```python
from build123d import *

# Parameters (mm, degrees)
EXTRUDE_6_DEPTH      = 4
CUT_EXTRUDE_12_DEPTH = 3
SKETCH_3_R           = 2.6
CUT_EXTRUDE_13_DEPTH = 4


with BuildPart() as part:
    # 草圖1 → 填料-伸長6 (new body)
    with BuildSketch(Plane(origin=(0, 0, 0), x_dir=(1, 0, 0), z_dir=(0, 1, 0))):
        with BuildLine():
            Line((0, 0), (0, 38.27))
            ThreePointArc((0, 38.27), (10, 48.27), (20, 38.27))
            Line((20, 38.27), (20, 0))
            Line((20, 0), (0, 0))
        make_face()
    extrude(amount=-EXTRUDE_6_DEPTH)

    # 草圖2 → 除料-伸長12 (cut)
    with BuildSketch(Plane(origin=(0, 0, 0), x_dir=(1, 0, 0), z_dir=(0, 1, 0))):
        with BuildLine():
            Line((7.4, 38.722411537), (5, 24.929659817))
            ThreePointArc((5, 24.929659817), (3.500000254, 20.778165453), (4.997678036, 16.625832861))
            Line((4.997678036, 16.625832861), (7.4, 2.833485375))
            ThreePointArc((7.4, 2.833485375), (10, 0.647203241), (12.6, 2.833485375))
            Line((12.6, 2.833485375), (15.002321964, 16.625832861))
            ThreePointArc((15.002321964, 16.625832861), (16.499999746, 20.778165453), (15, 24.929659817))
            Line((15, 24.929659817), (12.6, 38.722411537))
            ThreePointArc((12.6, 38.722411537), (10, 40.909067297), (7.4, 38.722411537))
        make_face()
    extrude(amount=-CUT_EXTRUDE_12_DEPTH, mode=Mode.SUBTRACT)

    # 草圖3 → 除料-伸長13 (cut)
    with BuildSketch(Plane(origin=(0, 0, 0), x_dir=(1, 0, 0), z_dir=(0, 1, 0))):
        with Locations((10, 20.776347886)):
            Circle(SKETCH_3_R)
    extrude(amount=-CUT_EXTRUDE_13_DEPTH, mode=Mode.SUBTRACT)


solid = part.part
```
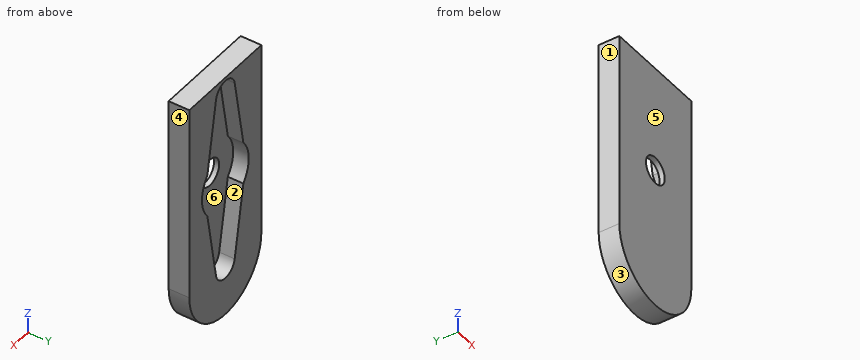
Geometry: final body of the model. Coordinates: model frame, mm. Face numbers are marked on the shaded views. A direction names the side the tool comes from. Coordinates: 2 decimals unless noted, no trailing zeros. Order: outer loops, then holes, each group sorted by start corner. A loop starts at its lowest first (then second) coordinate and runs counter-clockwise, first axis right, second up. Notation, with made-up numbers: M 42.25,41.5 L 89.25,41.5 A33 ccw 89.25,76.5 Z; hole C 12.25,-38.75 d11. An arc over 180 degrees is marked long. Answer in a Markdown table with one row per item. Add a question column.
Q1. Section query D-D on x = 14.25. Return the cut outline in (y, z).
Q2. Reachability of the marked faces 1 and 2 from +Z, -Z, +X, -X, +Y, -Y: full face, straight path, thin tool, end or side. Return the list, or none.
Q3. Section query A-A on x = 10. Return the cut outline in (y, z), and give its area (3 significant figures).
Q4. Section query B-B on y = -2.2. Return the cut outline in (x, z).
Q5. Mould query, pull axis X, two halves, no side actions, for the marked faces 3, 4, 5 and 6. Classes: released by +X, released by -X, zero draft, split by the parting line, or undercut.
Q6. Section query C-C on z = -12.5. Return the cut outline in (x, y), and give its area (3 significant figures).
Q7. Contact query for flat-ended pins moving along their axis: P1, Ø12, axis at x = 3.5, z = -38.5, coming from the +Y side; P2, Ø2, axis at x = 2.5, y = -1, coming from the -Z side; P3, Ø4, axis at x = 13, z = -23.5, coming from the +Y side. Output: stop coordinate, or through.
Q8. Line query: L1, parallel to Z at x = 10, y = -3.6; L2, parallel to X at y = -0.65, z = -20.5; L3, parallel to Y at x = 7.75, z = -7. Output: solid intervals per line, ascending.
Completed:
| question | item | result |
|---|---|---|
| 1 | outline | M -4,-47.32 L 0,-47.32 L 0,-29.24 L -3,-29.24 L -3,-12.31 L 0,-12.31 L 0,0 L -4,0 Z |
| 2 | face 1 | +Z, -Z, -X, +Y, -Y |
| 2 | face 2 | +Y |
| 3 | outline | M -4,-48.27 L 0,-48.27 L 0,-40.91 L -3,-40.91 L -3,-23.38 L -4,-23.38 Z; M -4,-18.18 L -3,-18.18 L -3,-0.65 L 0,-0.65 L 0,0 L -4,0 Z |
| 3 | area | 67.1 mm2 |
| 4 | outline | M 0,-38.27 A10 ccw 20,-38.27 L 20,0 L 0,0 Z; hole M 5,-24.93 L 7.4,-38.72 A2.64 ccw 12.6,-38.72 L 15,-24.93 A6.5 ccw 15,-16.63 L 12.6,-2.83 A2.64 ccw 7.4,-2.83 L 5,-16.63 A6.5 ccw Z |
| 5 | face 3 | split by the parting line |
| 5 | face 4 | released by +X |
| 5 | face 5 | zero draft |
| 5 | face 6 | undercut |
| 6 | outline | M 0,-4 L 20,-4 L 20,0 L 14.28,0 L 14.28,-3 L 5.72,-3 L 5.72,0 L 0,0 Z |
| 6 | area | 54.3 mm2 |
| 7 | P1 | stops at y = 0 |
| 7 | P2 | stops at z = -45.87 |
| 7 | P3 | stops at y = -3 |
| 8 | L1 | z = -48.27 to -23.38, -18.18 to 0 |
| 8 | L2 | x = 0 to 3.51, 16.49 to 20 |
| 8 | L3 | y = -4 to -3 |
